from build123d import *

# Parameters (mm, degrees)
ESQUISSE1_W             = 46
ESQUISSE1_H             = 46
ESQUISSE1_W_2           = 40
ESQUISSE1_H_2           = 40
BOSS_EXTRU_1_DEPTH      = 80
ESQUISSE2_W             = 46
ESQUISSE2_H             = 46
ESQUISSE2_W_2           = 40
ESQUISSE2_H_2           = 40
BOSS_EXTRU_2_DEPTH      = 40
BOSS_EXTRU_3_DEPTH      = 3
BOSS_EXTRU_4_DEPTH      = 3
ESQUISSE5_R             = 1.5
ENL_V_MAT_EXTRU_1_DEPTH = 104.111590037


with BuildPart() as part:
    # Esquisse1 → Boss.-Extru.1 (new body)
    with BuildSketch(Plane.XY):
        with Locations((23, -23)):
            Rectangle(ESQUISSE1_W, ESQUISSE1_H)
        with Locations((23, -23)):
            Rectangle(ESQUISSE1_W_2, ESQUISSE1_H_2, mode=Mode.SUBTRACT)
    extrude(amount=BOSS_EXTRU_1_DEPTH)

    # Esquisse2 → Boss.-Extru.2 (add)
    with BuildSketch(Plane(origin=(0, 0, 0), x_dir=(1, 0, 0), z_dir=(0, 1, 0))):
        with Locations((23, -23)):
            Rectangle(ESQUISSE2_W, ESQUISSE2_H)
        with Locations((23, -23)):
            Rectangle(ESQUISSE2_W_2, ESQUISSE2_H_2, mode=Mode.SUBTRACT)
    extrude(amount=BOSS_EXTRU_2_DEPTH)

    # Esquisse3 → Boss.-Extru.3 (add)
    with BuildSketch(Plane(origin=(46, 0, 0), x_dir=(0, 0, -1), z_dir=(1, 0, 0))):
        Polygon((-80, 0), (-46, 40), (-46, 0), align=None)
    extrude(amount=-BOSS_EXTRU_3_DEPTH)

    # Esquisse4 → Boss.-Extru.4 (add)
    with BuildSketch(Plane.ZY):
        Polygon((46, 40), (80, 0), (46, 0), align=None)
    extrude(amount=-BOSS_EXTRU_4_DEPTH)

    # Esquisse5 → Enlèv. mat.-Extru.1 (cut, through all)
    with BuildSketch(Plane.ZY):
        with Locations(Location((23, 20, 0), (0, 0, 270))):
            Circle(ESQUISSE5_R)
        with Locations(Location((20, -23, 0), (0, 0, 270))):
            Circle(ESQUISSE5_R)
        with Locations(Location((60, -23, 0), (0, 0, 270))):
            Circle(ESQUISSE5_R)
    extrude(amount=-ENL_V_MAT_EXTRU_1_DEPTH, mode=Mode.SUBTRACT)


solid = part.part
Work out the finished part from the listing and answer in its coordinate system (mm). A direction names the side the tool comes from. Round coordinates to 2 decimals unless told otherwise and drop trailing zeros. Loops run counter-clockwise (first coordinate to the right, second up) from the corner with the lowest first, then second, coordinate; pieces in that order, holes last. Notation, with made-up numbers: M 55,-3.5 L 94,-3.5 A21 ccw 94,20.5 Z; hole C -8,49 d11. An arc over 180 degrees is marked long. One line per question, with ' | ' between items. Start each with the question number.
(1) A cutting plane is placed at D-D on y = 10. Write down the section's boundary in (x, z).
(2) Flat-ended cylindrical pins translate along their axes: pin 1 Ø5 at (x, z) = (11, 56.5) entering from +Y; pin 2 Ø20 at (x, y) = (27.5, 24.5) entering from +Z. Find the tip coordinate at first contact, or state that the pin passes through.
(3) Find the intervals of material crossed by line 1 (Z direction, x = 1.2, y = -23); line 2 (Y direction, x = 25, z = 24); line 3 (X direction, y = -8.5, z = 17.5), in increasing order.
(4) A tool of negligible diameter and unlimited length cuts with its end or side. For faces 1 (the face through (23, -3, 39)), 2 (the face through (43, 20, 28)), 3 (the face through (23, 20, 46)), 4 (the face through (46, -2, 39)), from which of +Z, -Z, +X, -X, +Y, -Y can it reach the whole face along a straight path? Write none if from no direction.
(5) A cutting plane is placed at A-A on y = -9. Write down the section's boundary in (x, z).
(6) A cutting plane is placed at C-C on z = 23. Write down the section's boundary in (x, y), plus the area to 3 significant figures.
(7) A cutting plane is placed at B-B on x = 34.5. Write down the section's boundary in (y, z), plus the area to 3 significant figures.
(8) For a pull along Z with two mould halves and no side action, classify faces 5 (the face through (1, 20, 63)), 6 (the face through (23, 16, 0)), 7 (the face through (23, 20, 3)), 8 (the face through (23, -43, 39)) as released by +Z, released by -Z, zero draft, split by the parting line, or undercut.
Geometry check:
1) outline: M 0,0 L 46,0 L 46,71.5 L 43,71.5 L 43,46 L 3,46 L 3,71.5 L 0,71.5 Z; hole M 3,3 L 43,3 L 43,43 L 3,43 Z
2) pin 1: stops at y = 0 | pin 2: stops at z = 46
3) line 1: z = 0 to 18.5, 21.5 to 58.5, 61.5 to 80 | line 2: y = -46 to -43, -3 to 0 | line 3: x = 0 to 3, 43 to 46
4) face 1: +Z, -Z | face 2: +Y | face 3: +Z, +Y | face 4: +Z, -Z, +X, +Y, -Y
5) outline: M 0,0 L 3,0 L 3,80 L 0,80 Z; M 43,0 L 46,0 L 46,80 L 43,80 Z
6) outline: M 0,-46 L 46,-46 L 46,18.5 L 43,18.5 L 43,0 L 3,0 L 3,18.5 L 0,18.5 Z; M 0,21.5 L 3,21.5 L 3,40 L 0,40 Z; M 43,21.5 L 46,21.5 L 46,40 L 43,40 Z; hole M 3,-43 L 43,-43 L 43,-3 L 3,-3 Z | area: 738 mm²
7) outline: M -46,0 L -43,0 L -43,80 L -46,80 Z; M -3,0 L 40,0 L 40,3 L 0,3 L 0,43 L 40,43 L 40,46 L 0,46 L 0,80 L -3,80 Z | area: 720 mm²
8) face 5: released by +Z | face 6: released by -Z | face 7: undercut | face 8: zero draft
